Can you work these out from the model? Positions are in its coordinate system, mm. Face numbers are marked on the shaded views. A direction names the side the tool comes from. Give positions to 0.01 mm unless a question says otherwise; leave off trailing zeros. Loops run counter-clockwise (first coordinate to the right, second up) from the corner with the lowest first, then second, coordinate; pieces in that order, holes last. Notation, with made-up numbers: (36.5, 45) - (48.5, 45) arc R22 cw to (48.5, 59) - close; hole circle Ø8 at (6, 61.5). An arc over 180 degrees is marked (long way). Answer as a JSON object with one key per item and string values.
Autodesk Fusion 360 part; units mm, degrees
sketch "Sketch1" plane through (0, 0, 0) normal (0, 0, 1) x (1, 0, 0)
  circle A0 centre (0, 0) radius 17.65
  circle A1 centre (0, 0) radius 38
  circle A2 centre (0, 0) radius 50
  dimension "d1" = 35.3
  dimension "d2" = 76
  dimension "d3" = 100
extrude "Extrude1" add sketch "Sketch1" along normal blind 5 contours A1
extrude "Extrude2" add sketch "Sketch1" along normal blind 15 contours A2
sketch "Sketch2" plane through (0, 0, 5) normal (0, 0, 1) x (-1, 0, 0)
  circle A0 centre (0, 0) radius 17.65
  circle A1 centre (0, 0) radius 38
  circle A2 centre (0, 0) radius 22.5
  dimension "d8" = 45
extrude "Extrude3" add sketch "Sketch2" along normal blind 6 contours A2
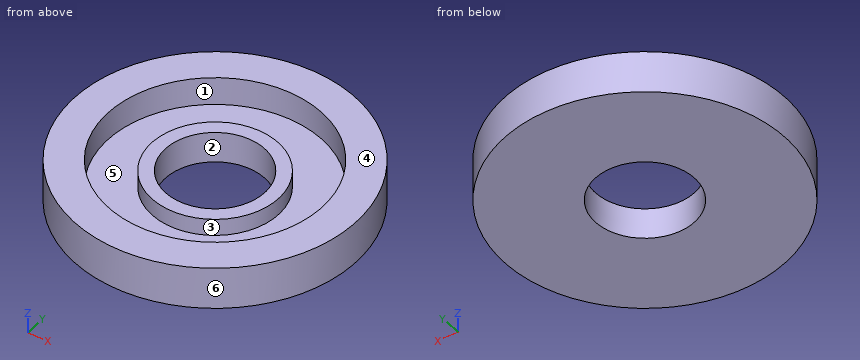
1) Imagine slicing it at A-A on y = 0. Write out the boundary of the cut face in (x, z).
Check sheet entries:
{"outline": "(-50, 0) - (-17.65, 0) - (-17.65, 11) - (-22.5, 11) - (-22.5, 5) - (-38, 5) - (-38, 15) - (-50, 15) - close; (17.65, 0) - (50, 0) - (50, 15) - (38, 15) - (38, 5) - (22.5, 5) - (22.5, 11) - (17.65, 11) - close"}
2) Which directions (+Z, -Z, +X, -X, +Y, -Y) give clear straight access to the entire face, cutting with the end or side of a thin tool? Please do the marked faces 1 and 2.
Check sheet entries:
{"face 1": "+Z", "face 2": "+Z, -Z"}
3) Imagine slicing it at C-C on z = 13.5. Write out the boundary of the cut face in (x, y), and give its area (3 significant figures).
Check sheet entries:
{"outline": "circle Ø100 at (0, 0); hole circle Ø76 at (0, 0)", "area": "3,320 mm2"}
4) If we mould it in two halves opening along X, with no side actions, what happens to the marked faces 3, 4, 5 and 6? For each: released by +X, released by -X, zero draft, split by the parting line, or undercut.
Check sheet entries:
{"face 3": "undercut", "face 4": "zero draft", "face 5": "undercut", "face 6": "split by the parting line"}
5) I need wall thicknesses on L1, parallel to Y at x = 0, z = 8.75; L2, parallel to Y at x = -15.5, z = 9.25; L3, parallel to Y at x = 0, z = 12.25. Which ranges of each line are inside material? Lowest first, please.
Check sheet entries:
{"L1": "-50 to -38, -22.5 to -17.65, 17.65 to 22.5, 38 to 50", "L2": "-47.54 to -34.7, -16.31 to -8.44, 8.44 to 16.31, 34.7 to 47.54", "L3": "-50 to -38, 38 to 50"}
6) Imagine slicing it at D-D on y = -36. Write out the boundary of the cut face in (x, z).
Check sheet entries:
{"outline": "(-34.7, 0) - (34.7, 0) - (34.7, 15) - (12.17, 15) - (12.17, 5) - (-12.17, 5) - (-12.17, 15) - (-34.7, 15) - close"}
7) I'm going to push flat-ended pins straight in: P1, Ø22.5, axis at x = 4, y = -8, coming from the +Z side; P2, Ø2, axis at y = 35, z = 1.5, coming from the -X side; P3, Ø5, axis at y = 37.5, z = 10, coming from the -X side. Where does each tip first touch, or does it pass through?
Check sheet entries:
{"P1": "z = 11", "P2": "x = -36.66", "P3": "x = -35.71"}
